Verification items for the finished model (mm, model axes). Give positions to 0.01 mm unless a question says otherwise; leave off trailing zeros. Write each loop counter-clockwise with the first axis right and the second up, starting at its lowest first coordinate (ties: lowest second). Pieces come first, ordered by that corner, then holes. Notation, with made-up numbers: (46.25, 6) -> (76.25, 6) arc R14 ccw to (76.25, 27) -> close; hole circle Ø10 at (49, 6.5). An arc over 180 degrees is marked (long way). Write item = value, one per line.
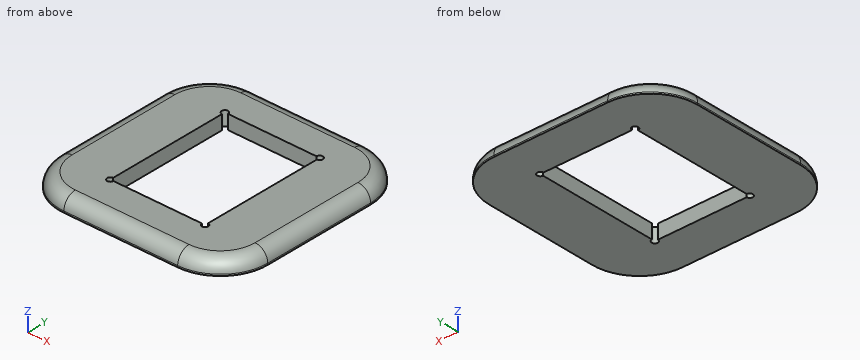
from build123d import *

# Parameters (mm, degrees)
F0_W     = 66.1
F0_H     = 66.1
F0_W_2   = 30.1
F0_H_2   = 40.2
F1_DEPTH = 4.5
F2_R     = 15
F3_R     = 4
F4_R     = 1
F5_DEPTH = 25


with BuildPart() as f1:
    # F0 (on Top) → F1 (new body)
    with BuildSketch(Plane.XY):
        Rectangle(F0_W, F0_H)
        Rectangle(F0_W_2, F0_H_2, mode=Mode.SUBTRACT)
    extrude(amount=F1_DEPTH)

    # F2
    f2_edges = [f1.edges().sort_by_distance(p)[0] for p in [
        (-33.05, -33.05, 2.25),
        (33.05, -33.05, 2.25),
        (-33.05, 33.05, 2.25),
        (33.05, 33.05, 2.25),
    ]]
    fillet(f2_edges, radius=F2_R)

    # F3
    f3_edges = [f1.edges().sort_by_distance(p)[0] for p in [
        (-28.656602, 28.656602, 4.5),
    ]]
    fillet(f3_edges, radius=F3_R)

    # F4 (on face) → F5 (cut)
    with BuildSketch(Plane.XY.offset(4.5)):
        with Locations((15.05, 20.1)):
            Circle(F4_R)
        with Locations((15.05, -20.1)):
            Circle(F4_R)
        with Locations((-15.05, -20.1)):
            Circle(F4_R)
        with Locations((-15.05, 20.1)):
            Circle(F4_R)
    extrude(amount=-F5_DEPTH, mode=Mode.SUBTRACT)


solid = f1.part
Item 1: Go/stop test with flat-tipped pins: P1, Ø1.8, axis at x = -15.05, y = -20.1, coming from the +Z side; P2, Ø2, axis at y = -0.5, z = 2, coming from the +X side; P3, Ø2, axis at x = -5.5, z = 2.5, coming from the +Y side. Record where each tip stops, or that it passes through.
Response values:
P1 = through
P2 = 33.02
P3 = 32.92
Item 2: Sectioned sample at B-B on z = 2.9. Record the cut outline in (x, y), then the cut area to 3 significant figures.
Response values:
outline = (-32.25, -18.05) arc R14.2 ccw to (-18.05, -32.25) -> (18.05, -32.25) arc R14.2 ccw to (32.25, -18.05) -> (32.25, 18.05) arc R14.2 ccw to (18.05, 32.25) -> (-18.05, 32.25) arc R14.2 ccw to (-32.25, 18.05) -> close; hole (-15.05, -19.1) arc R1 ccw (long way) to (-14.05, -20.1) -> (14.05, -20.1) arc R1 ccw (long way) to (15.05, -19.1) -> (15.05, 19.1) arc R1 ccw (long way) to (14.05, 20.1) -> (-14.05, 20.1) arc R1 ccw (long way) to (-15.05, 19.1) -> close
area = 2,770 mm^2
Item 3: Material ranges on line 1 (X direction, y = -8, z = 1.6); line 2 (Y direction, x = 5.5, z = 3.25); line 3 (X direction, y = 7.5, z = 2.55), recorded low to high.
Response values:
line_1 = -32.9 to -15.05, 15.05 to 32.9
line_2 = -31.95 to -20.1, 20.1 to 31.95
line_3 = -32.48 to -15.05, 15.05 to 32.48
Item 4: Sectioned sample at C-C on y = 14.5. Record the cut outline in (x, z).
Response values:
outline = (-33.05, 0) -> (-15.05, 0) -> (-15.05, 4.5) -> (-29.05, 4.5) arc R4 ccw to (-33.05, 0.5) -> close; (15.05, 0) -> (33.05, 0) -> (33.05, 0.5) arc R4 ccw to (29.05, 4.5) -> (15.05, 4.5) -> close
Item 5: Sectioned sample at A-A on x = 3.5. Record the cut outline in (y, z), then the cut area to 3 significant figures.
Response values:
outline = (-33.05, 0) -> (-20.1, 0) -> (-20.1, 4.5) -> (-29.05, 4.5) arc R4 ccw to (-33.05, 0.5) -> close; (20.1, 0) -> (33.05, 0) -> (33.05, 0.5) arc R4 ccw to (29.05, 4.5) -> (20.1, 4.5) -> close
area = 110 mm^2
